The drawing under review shows one solid part. Ordinate dimensions are in mm from its lowest x, y, z. A direction names the side the tool comes from. Coordinates: 2 decimals unless noted, no trailing zeros. Order: outer loops, then holes, each group sorted by start corner. A loop starts at its lowest first (then second) coordinate and runs counter-clockwise, first axis right, second up. Notation, with made-up numbers: (21, 59) -> (50, 59) arc R24 ccw to (50, 96) -> close; hole circle Ø2 at (-28, 49). An arc over 180 degrees is marked (long way). Use one line per item in the form item = value.
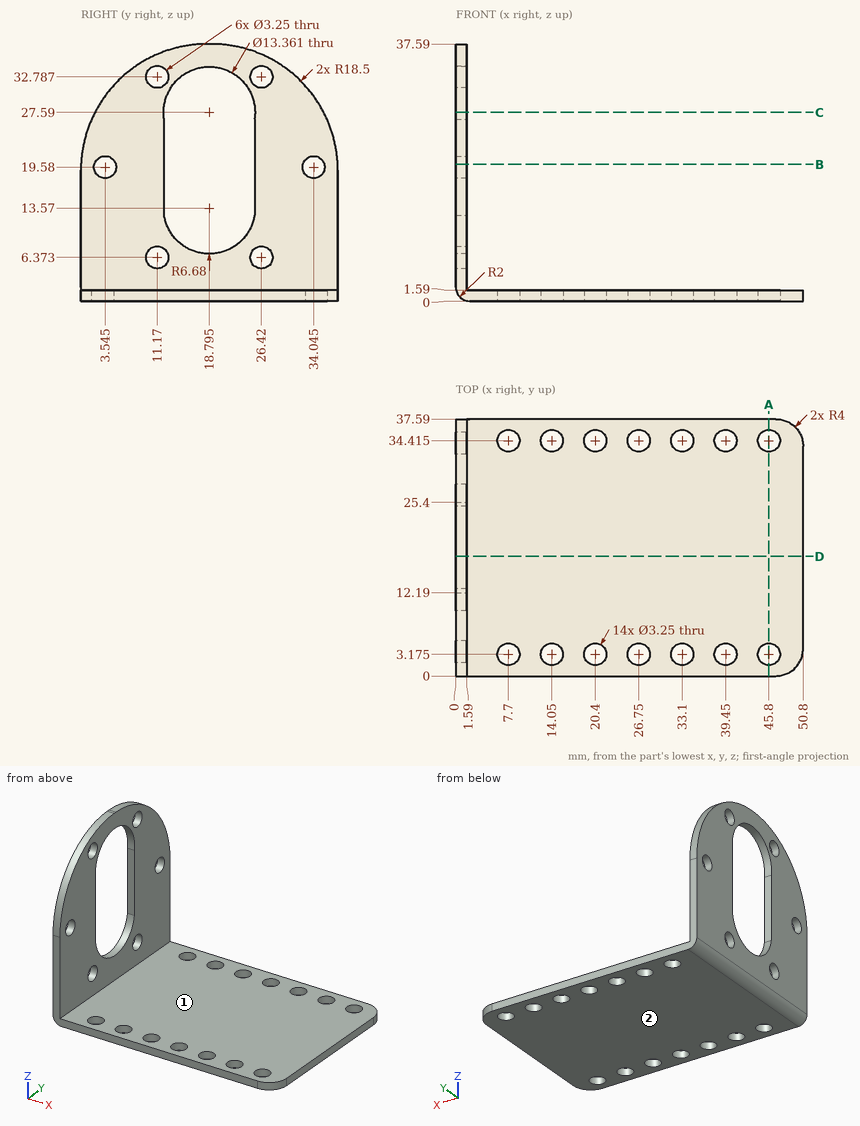
Item 1: To check wall thickness, follow L1, parallel to Y at x = 33.1, z = 1.2; L2, parallel to Y at x = 1.25, z = 19.58; L3, parallel to Z at x = 43.5, y = 26. State the ranges of each line that lie inside material, in increasing order. Write a range as from..to.
Results found:
L1 = 0..1.55, 4.8..32.79, 36.04..37.59
L2 = 0.01..1.92, 5.17..12.19, 25.4..32.42, 35.67..37.58
L3 = 0..1.59
Item 2: We need section A-A (x = 45.8). Write out the cut boundary in (y, z).
Results found:
outline = (0, 0) -> (1.55, 0) -> (1.55, 1.59) -> (0, 1.59) -> close; (4.8, 0) -> (32.79, 0) -> (32.79, 1.59) -> (4.8, 1.59) -> close; (36.04, 0) -> (37.59, 0) -> (37.59, 1.59) -> (36.04, 1.59) -> close
Item 3: Tool access review of the marked faces 1 and 2: name each direction out of +Z, -Z, +X, -X, +Y, -Y from which nothing blocks a thin tool from reaching the whole face with its end or side.
Results found:
face_1 = +Z, +X, +Y, -Y
face_2 = -Z, +X, -X, +Y, -Y
Item 4: Clearance check with flat-ended pins moving along their axes: pin 1 (5 mm diameter, centred on y = 26.42, z = 32.79, fed in from +X); pin 2 (3.5 mm diameter, centred on x = 33.1, y = 3.175, fed in from +Z). State where each tip first meets the part, or that it passes through.
Results found:
pin_1 = 1.59
pin_2 = 1.59
Item 5: We need section D-D (y = 17.5). Write out the cut boundary in (x, z).
Results found:
outline = (0, 2) arc R2 ccw to (2, 0) -> (50.8, 0) -> (50.8, 1.59) -> (1.59, 1.59) -> (1.59, 7.02) -> (0, 7.02) -> close; (0, 34.14) -> (1.59, 34.14) -> (1.59, 37.56) -> (0, 37.56) -> close
Item 6: We need section C-C (z = 27.59). Write out the cut boundary in (x, y) (1 decimal).
Results found:
outline = (0, 2.1) -> (1.6, 2.1) -> (1.6, 12.1) -> (0, 12.1) -> close; (0, 25.5) -> (1.6, 25.5) -> (1.6, 35.5) -> (0, 35.5) -> close
Item 7: We need section B-B (z = 20). Write out the cut boundary in (x, y) (1 decimal).
Results found:
outline = (0, 0) -> (1.6, 0) -> (1.6, 2) -> (0, 2) -> close; (0, 5.1) -> (1.6, 5.1) -> (1.6, 12.2) -> (0, 12.2) -> close; (0, 25.4) -> (1.6, 25.4) -> (1.6, 32.5) -> (0, 32.5) -> close; (0, 35.6) -> (1.6, 35.6) -> (1.6, 37.6) -> (0, 37.6) -> close
